```python
from build123d import *

# Parameters (mm, degrees)
SKETCH1_W               = 60
SKETCH1_H               = 30
BOSS_EXTRUDE1_DEPTH     = 50
CUT_EXTRUDE1_DEPTH      = 50
CUT_EXTRUDE2_DEPTH      = 61.207972894
CUT_EXTRUDE2_DEPTH_BACK = 61.207972894
CUT_EXTRUDE4_DEPTH      = 61.207972894
CUT_EXTRUDE4_DEPTH_BACK = 61.207972894
SKETCH5_R               = 3


with BuildPart() as part:
    # Sketch1 → Boss-Extrude1 (new body)
    with BuildSketch(Plane.XY):
        Rectangle(SKETCH1_W, SKETCH1_H)
    extrude(amount=BOSS_EXTRUDE1_DEPTH)

    # Sketch2 → Cut-Extrude1 (cut)
    with BuildSketch(Plane.XY.offset(50)):
        Polygon((-30, 9), (0, 15), (-30, 15), align=None)
        Polygon((30, 15), (0, 15), (30, 9), align=None)
        Polygon((0, -15), (-30, -9), (-30, -15), align=None)
        Polygon((30, -15), (30, -9), (0, -15), align=None)
    extrude(amount=-CUT_EXTRUDE1_DEPTH, mode=Mode.SUBTRACT)

    # Sketch4 → Cut-Extrude2 (cut, two sides: drawn at the far end of the back side and taken through both)
    with BuildSketch(Plane(origin=(0, 0, 0), x_dir=(1, 0, 0), z_dir=(0, 1, 0)).offset(-CUT_EXTRUDE2_DEPTH_BACK)):
        Polygon((-30, 0), (0, 0), (-30, -8), align=None)
        Polygon((30, 0), (30, -8), (0, 0), align=None)
        Polygon((30, -50), (0, -50), (30, -42), align=None)
        Polygon((-30, -42), (-30, -50), (0, -50), align=None)
    extrude(amount=CUT_EXTRUDE2_DEPTH + CUT_EXTRUDE2_DEPTH_BACK, mode=Mode.SUBTRACT)

    # Sketch5 → Cut-Extrude4 (cut, two sides: drawn at the far end of the back side and taken through both)
    with BuildSketch(Plane.XY.offset(-CUT_EXTRUDE4_DEPTH_BACK)):
        with Locations((-24, 0)):
            Circle(SKETCH5_R)
        with Locations((24, 0)):
            Circle(SKETCH5_R)
    extrude(amount=CUT_EXTRUDE4_DEPTH + CUT_EXTRUDE4_DEPTH_BACK, mode=Mode.SUBTRACT)


solid = part.part
```
The listing builds one solid part. Answer for the finished solid, in the listing's coordinates (mm). Give positions to 0.01 mm unless a question says otherwise; leave off trailing zeros. Loops run counter-clockwise (first coordinate to the right, second up) from the corner with the lowest first, then second, coordinate; pieces in that order, holes last. Notation, with made-up numbers: M 22,45.25 L 81,45.25 A36 cw 81,81.25 Z; hole C -28,74 d11. An arc over 180 degrees is marked long. One line per item, written item: value.
1. Section D-D on y = 6 is taken. Determine the outline of the cut face in (x, z), plus the area to 3 significant figures.
Found:
outline: M -30,8 L 0,0 L 30,8 L 30,42 L 0,50 L -30,42 Z
area: 2,520 mm^2
2. Section C-C on z = 27.5 is taken. Determine the outline of the cut face in (x, y), plus the area to 3 significant figures.
Found:
outline: M -30,-9 L 0,-15 L 30,-9 L 30,9 L 0,15 L -30,9 Z; hole C -24,0 d6; hole C 24,0 d6
area: 1,380 mm^2
3. Each of these flat-tipped pins is pushed along its axis until it touches: P1, Ø1.5, axis at x = 13.5, y = 12, coming from the +Z side; P2, Ø3, axis at x = -12.5, z = 13, coming from the -Y side; P3, Ø5, axis at x = 0.5, z = 27, coming from the +Y side; P4, Ø1.5, axis at x = -22, z = 26.5, coming from the +Y side. Where does it stop, or does it pass through?
Found:
P1: z = 46.6
P2: y = -12.8
P3: y = 15
P4: y = 10.75
4. Find the intervals of material crossed by probe 1 along X at (y, z) = (0, 16); probe 2 along X at (y, z) = (1, 16.5); probe 3 along Y at (x, z) = (-24, 22), in increasing order.
Found:
probe 1: -30 to -27, -21 to 21, 27 to 30
probe 2: -30 to -26.83, -21.17 to 21.17, 26.83 to 30
probe 3: -10.2 to -3, 3 to 10.2
5. For a pull along Y with two mould halves and no side action, classify faces 1 (the face through (21, 0, 25)), 2 (the face through (-11.457, -0.21, 46.945)), 3 (the face through (15, 12, 25)) as pulls with the +Y half, pulls with the -Y half, needs draft (parallel to the pull), parting line crosses it, or undercut.
Found:
face 1: undercut
face 2: needs draft
face 3: pulls with the +Y half
6. Section B-B on x = -24 is taken. Determine the outline of the cut face in (y, z).
Found:
outline: M -10.2,6.4 L -3,6.4 L -3,43.6 L -10.2,43.6 Z; M 3,6.4 L 10.2,6.4 L 10.2,43.6 L 3,43.6 Z
7. Section A-A on y = 0 is taken. Determine the outline of the cut face in (x, z), plus the area to 3 significant figures.
Found:
outline: M -30,8 L -27,7.2 L -27,42.8 L -30,42 Z; M -21,5.6 L 0,0 L 21,5.6 L 21,44.4 L 0,50 L -21,44.4 Z; M 27,7.2 L 30,8 L 30,42 L 27,42.8 Z
area: 2,070 mm^2
